Check sheet for the drawn part. Datum: minimum x, y, z corner. Units: mm. Give positions to 0.01 mm unless a question says otherwise; leave off trailing zeros. Loops run counter-clockwise (first coordinate to the right, second up) from the corner with the lowest first, then second, coordinate; pieces in that order, holes last. Notation, with made-up numbers: (-32, -19.5) - (-9, -19.5) arc R16 ccw to (-9, 3.5) - close; hole circle Ø10 at (10, 19). An arc over 180 degrees is marked (long way). Use a Markdown table: item, result. Add a question column.
1. Cross-section at B-B on x = 70.5. Enter the section's corners in (y, z).
2. Cross-section at C-C on y = 75. Enter the section's corners in (x, z) (1 decimal), and give its area (3 significant figures).
3. Draft check along Z on the marked faces 1, 2 and 3. Enter one of: pulls with the +Z half, pulls with the -Z half, needs draft (parallel to the pull), parting line crosses it, or undercut.
4. Cross-section at D-D on x = 105. Enter the section's corners in (y, z).
5. Cross-section at A-A on z = 96. Enter the section's corners in (x, y).
6. Material ranges on L1, parallel to Z at x = 59, y = 75; L2, parallel to X at y = 107, z = 83 (1 decimal); L3, parallel to Z at x = 83.5, y = 79, recorded low to high.
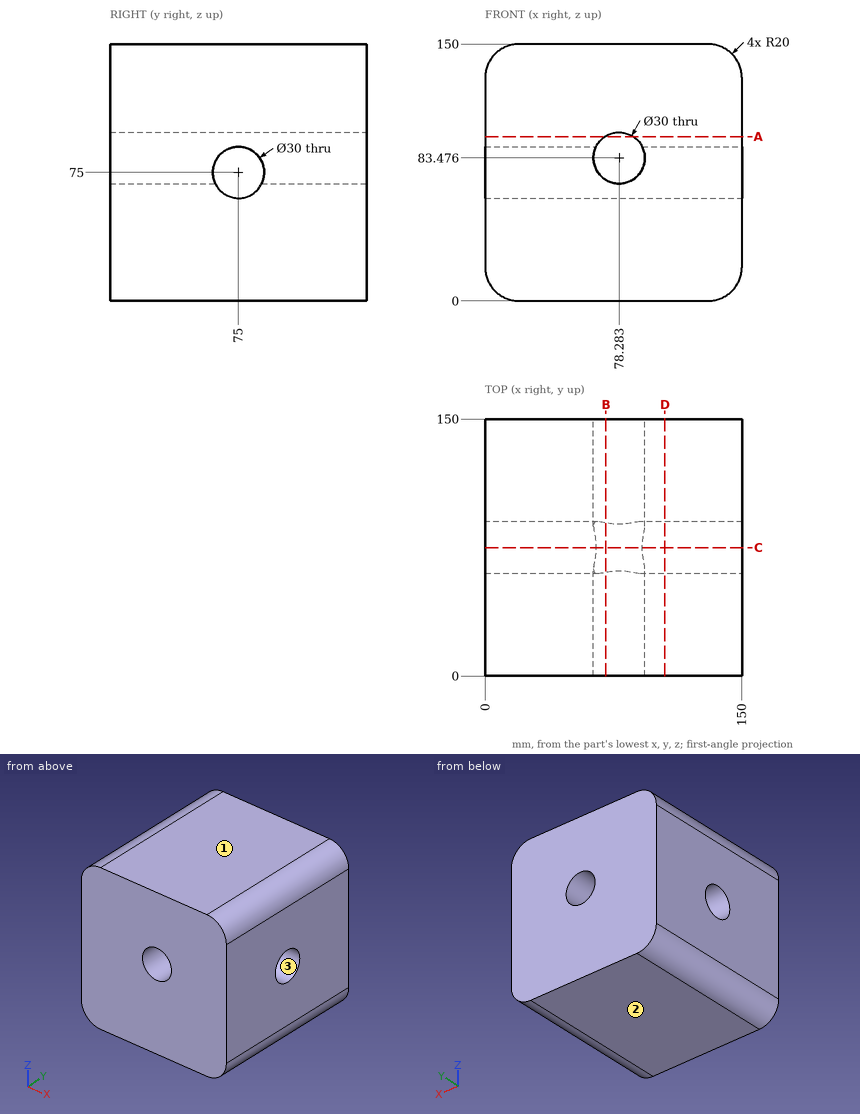
Values found:
| question | item | result |
|---|---|---|
| 1 | outline | (0, 0) - (150, 0) - (150, 70.65) - (89.36, 70.65) arc R15 cw to (60.64, 70.65) - (0, 70.65) - close; (0, 96.3) - (150, 96.3) - (150, 150) - (0, 150) - close |
| 2 | outline | (0, 20) arc R20 ccw to (20, 0) - (130, 0) arc R20 ccw to (150, 20) - (150, 60) - (0, 60) - close; (0, 90) - (64.8, 90) arc R15 cw to (91.8, 90) - (150, 90) - (150, 130) arc R20 ccw to (130, 150) - (20, 150) arc R20 ccw to (0, 130) - close |
| 2 | area | 17,500 mm2 |
| 3 | face 1 | pulls with the +Z half |
| 3 | face 2 | pulls with the -Z half |
| 3 | face 3 | undercut |
| 4 | outline | (0, 0) - (150, 0) - (150, 150) - (0, 150) - close; hole circle Ø30 at (75, 75) |
| 5 | outline | (0, 0) - (70.03, 0) - (70.03, 150) - (0, 150) - close; (86.54, 0) - (150, 0) - (150, 150) - (86.54, 150) - close |
| 6 | L1 | z = 0 to 60, 90 to 150 |
| 6 | L2 | x = 0 to 63.3, 93.3 to 150 |
| 6 | L3 | z = 0 to 60.54, 97.54 to 150 |
